Can you work these out from the model? Positions are in its coordinate system, mm. Give positions to 0.01 mm unless a question says otherwise; leave off trailing zeros. Return JSON: item names as keys, results as strings. Group by question number.
Q1. Will these pins go through, and if not, where does the flat tip stop? pin 1 (9 mm diameter, centred on x = 14.29, z = -609.6, fed in from +Y); pin 2 (4 mm diameter, centred on x = 138.11, z = -1168.4, fed in from -Y) (1 decimal); pin 3 (11 mm diameter, centred on x = 138.11, z = -609.6, fed in from +Y); pin 4 (2 mm diameter, centred on y = 3, z = -487.5, fed in from -X).
Q2. I need wall thicknesses on line 1 along X through (y, z) = (0.85, -609.6); line 2 along Z through (x, y) = (14.5, 5); line 3 along X through (y, z) = (2.05, -50.8). Which ranges of each line are inside material? Lowest first, please. Write a range as [from, to].
Q3. Suppose I cut it at B-B, the plane y = 5.25. Count the separate pieces of the cut face and the enclosed holes in it, and give its area (3 significant figures).
```python
from build123d import *

# Parameters (mm, degrees)
SKETCH1_W                                     = 152.4
SKETCH1_H                                     = 1219.2
BOSS_EXTRUDE1_DEPTH                           = 6.35
CSK_FOR_1_4_FLAT_HEAD_MACHINE_SCREW1_AT_COUNT = 2
CSK_FOR_1_4_FLAT_HEAD_MACHINE_SCREW1_AT_PITCH = 123.825
CSK_FOR_1_4_FLAT_HEAD_MACHINE_SCREW1_2_COUNT  = 2
CSK_FOR_1_4_FLAT_HEAD_MACHINE_SCREW1_2_PITCH  = 305.609212271
CSK_FOR_1_4_FLAT_HEAD_MACHINE_SCREW1_3_COUNT  = 2
CSK_FOR_1_4_FLAT_HEAD_MACHINE_SCREW1_3_PITCH  = 572.354846773
CSK_FOR_1_4_FLAT_HEAD_MACHINE_SCREW1_4_COUNT  = 2
CSK_FOR_1_4_FLAT_HEAD_MACHINE_SCREW1_4_PITCH  = 847.296801968
CSK_FOR_1_4_FLAT_HEAD_MACHINE_SCREW1_5_COUNT  = 2
CSK_FOR_1_4_FLAT_HEAD_MACHINE_SCREW1_5_PITCH  = 1124.438700252
CSK_FOR_1_4_FLAT_HEAD_MACHINE_SCREW1_6_COUNT  = 2
CSK_FOR_1_4_FLAT_HEAD_MACHINE_SCREW1_6_PITCH  = 279.4
CSK_FOR_1_4_FLAT_HEAD_MACHINE_SCREW1_7_COUNT  = 2
CSK_FOR_1_4_FLAT_HEAD_MACHINE_SCREW1_7_PITCH  = 558.8
CSK_FOR_1_4_FLAT_HEAD_MACHINE_SCREW1_8_COUNT  = 2
CSK_FOR_1_4_FLAT_HEAD_MACHINE_SCREW1_8_PITCH  = 838.2
CSK_FOR_1_4_FLAT_HEAD_MACHINE_SCREW1_9_COUNT  = 2
CSK_FOR_1_4_FLAT_HEAD_MACHINE_SCREW1_9_PITCH  = 1117.6
CHAMFER1_SIZE                                 = 6.35


with BuildPart() as part:
    # Sketch1 → Boss-Extrude1 (new body)
    with BuildSketch(Plane(origin=(0, 0, 0), x_dir=(1, 0, 0), z_dir=(0, 1, 0))):
        with Locations((76.2, 609.6)):
            Rectangle(SKETCH1_W, SKETCH1_H)
    extrude(amount=BOSS_EXTRUDE1_DEPTH)

    # Sketch3 → CSK for 1/4 Flat Head Machine Screw1 (revolve, cut)
    with BuildSketch(Plane(origin=(14.2875, 6.35, -1168.4), x_dir=(0, 0, 1), z_dir=(1, 0, 0))):
        Polygon((0, 0), (0, 6.35), (3.3782, 6.35), (3.3782, 3.520932584), (6.4389, 0), align=None)
    csk_for_1_4_flat_head_machine_screw1 = revolve(axis=Axis((14.2875, 12.7, -1168.4), (0, -1, 0)), mode=Mode.SUBTRACT)

    # CSK for 1/4 Flat Head Machine Screw1 at: CSK for 1/4 Flat Head Machine Screw1 ×2
    with Locations(*[(i * CSK_FOR_1_4_FLAT_HEAD_MACHINE_SCREW1_AT_PITCH, 0, 0) for i in range(1, CSK_FOR_1_4_FLAT_HEAD_MACHINE_SCREW1_AT_COUNT)]):
        add(csk_for_1_4_flat_head_machine_screw1, mode=Mode.SUBTRACT)

    # CSK for 1_4 Flat Head Machine Screw1 2: CSK for 1/4 Flat Head Machine Screw1 ×2
    with Locations(*[Vector(0.405174304399354, 0, 0.9142394560805718) * (i * CSK_FOR_1_4_FLAT_HEAD_MACHINE_SCREW1_2_PITCH) for i in range(1, CSK_FOR_1_4_FLAT_HEAD_MACHINE_SCREW1_2_COUNT)]):
        add(csk_for_1_4_flat_head_machine_screw1, mode=Mode.SUBTRACT)

    # CSK for 1_4 Flat Head Machine Screw1 3: CSK for 1/4 Flat Head Machine Screw1 ×2
    with Locations(*[Vector(0.21634306182267615, 0, 0.9763174071997232) * (i * CSK_FOR_1_4_FLAT_HEAD_MACHINE_SCREW1_3_PITCH) for i in range(1, CSK_FOR_1_4_FLAT_HEAD_MACHINE_SCREW1_3_COUNT)]):
        add(csk_for_1_4_flat_head_machine_screw1, mode=Mode.SUBTRACT)

    # CSK for 1_4 Flat Head Machine Screw1 4: CSK for 1/4 Flat Head Machine Screw1 ×2
    with Locations(*[Vector(0.1461412337594335, 0, 0.9892637362176331) * (i * CSK_FOR_1_4_FLAT_HEAD_MACHINE_SCREW1_4_PITCH) for i in range(1, CSK_FOR_1_4_FLAT_HEAD_MACHINE_SCREW1_4_COUNT)]):
        add(csk_for_1_4_flat_head_machine_screw1, mode=Mode.SUBTRACT)

    # CSK for 1_4 Flat Head Machine Screw1 5: CSK for 1/4 Flat Head Machine Screw1 ×2
    with Locations(*[Vector(0.11012160998392527, 0, 0.9939181208804618) * (i * CSK_FOR_1_4_FLAT_HEAD_MACHINE_SCREW1_5_PITCH) for i in range(1, CSK_FOR_1_4_FLAT_HEAD_MACHINE_SCREW1_5_COUNT)]):
        add(csk_for_1_4_flat_head_machine_screw1, mode=Mode.SUBTRACT)

    # CSK for 1_4 Flat Head Machine Screw1 6: CSK for 1/4 Flat Head Machine Screw1 ×2
    with Locations(*[(0, 0, i * CSK_FOR_1_4_FLAT_HEAD_MACHINE_SCREW1_6_PITCH) for i in range(1, CSK_FOR_1_4_FLAT_HEAD_MACHINE_SCREW1_6_COUNT)]):
        add(csk_for_1_4_flat_head_machine_screw1, mode=Mode.SUBTRACT)

    # CSK for 1_4 Flat Head Machine Screw1 7: CSK for 1/4 Flat Head Machine Screw1 ×2
    with Locations(*[(0, 0, i * CSK_FOR_1_4_FLAT_HEAD_MACHINE_SCREW1_7_PITCH) for i in range(1, CSK_FOR_1_4_FLAT_HEAD_MACHINE_SCREW1_7_COUNT)]):
        add(csk_for_1_4_flat_head_machine_screw1, mode=Mode.SUBTRACT)

    # CSK for 1_4 Flat Head Machine Screw1 8: CSK for 1/4 Flat Head Machine Screw1 ×2
    with Locations(*[(0, 0, i * CSK_FOR_1_4_FLAT_HEAD_MACHINE_SCREW1_8_PITCH) for i in range(1, CSK_FOR_1_4_FLAT_HEAD_MACHINE_SCREW1_8_COUNT)]):
        add(csk_for_1_4_flat_head_machine_screw1, mode=Mode.SUBTRACT)

    # CSK for 1_4 Flat Head Machine Screw1 9: CSK for 1/4 Flat Head Machine Screw1 ×2
    with Locations(*[(0, 0, i * CSK_FOR_1_4_FLAT_HEAD_MACHINE_SCREW1_9_PITCH) for i in range(1, CSK_FOR_1_4_FLAT_HEAD_MACHINE_SCREW1_9_COUNT)]):
        add(csk_for_1_4_flat_head_machine_screw1, mode=Mode.SUBTRACT)

    # Chamfer1
    chamfer1_edges = [part.edges().sort_by_distance(p)[0] for p in [
        (0, 6.35, -609.6),
        (152.4, 6.35, -609.6),
    ]]
    chamfer(chamfer1_edges, length=CHAMFER1_SIZE - 0.0001)  # a hair under: the kernel refuses the full size


solid = part.part
```
Ans:
{
 "1": {"pin 1": "stops at y = 4.12", "pin 2": "passes through", "pin 3": "stops at y = 5.27", "pin 4": "stops at x = 2"},
 "2": {"line 1": "x = [0.85, 10.91], [17.67, 134.73], [141.49, 151.55]", "line 2": "z = [-1219.2, -1173.66], [-1163.14, -894.26], [-883.74, -614.86], [-604.34, -335.46], [-324.94, -56.06], [-45.54, 0]", "line 3": "x = [2.05, 10.91], [17.67, 134.73], [141.49, 150.35]"},
 "3": {"separate pieces": "1", "enclosed holes": "10", "area": "172,000 mm^2"}
}
